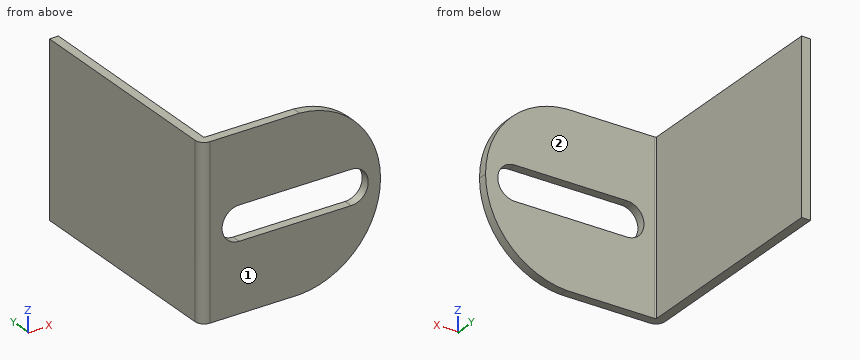
```python
from build123d import *

# Parameters (mm, degrees)
SKETCH1_W           = 19
SKETCH1_H           = 2
BOSS_EXTRUDE1_DEPTH = 38
CUT_EXTRUDE1_DEPTH  = 38


with BuildPart() as part:
    # Sketch1 → Boss-Extrude1 (new body)
    with BuildSketch(Plane.XY):
        with BuildLine():
            ThreePointArc((-18.000000186, -22.8), (-17.941421543, -22.941421356), (-17.800000186, -23))
            Line((-17.800000186, -23), (1.000000186, -23))
            Line((1.000000186, -23), (1.000000186, -25))
            Line((1.000000186, -25), (-18.000000186, -25))
            ThreePointArc((-18.000000186, -25), (-19.414213749, -24.414213562), (-20.000000186, -23))
            Line((-20.000000186, -23), (-20.000000186, 23))
            Line((-20.000000186, 23), (-20.000000186, 25))
            Line((-20.000000186, 25), (-18.000000186, 25))
            Line((-18.000000186, 25), (-18.000000186, 23))
            Line((-18.000000186, 23), (-18.000000186, -22.8))
        make_face()
        with Locations((10.500000186, -24)):
            Rectangle(SKETCH1_W, SKETCH1_H)
    extrude(amount=BOSS_EXTRUDE1_DEPTH)

    # Sketch2 → Cut-Extrude1 (cut)
    with BuildSketch(Plane.XZ.offset(25)):
        with BuildLine():
            Line((20.000000186, 0), (20.000000186, 19))
            ThreePointArc((20.000000186, 19), (14.768114469, 5.896541545), (1.950000354, 0))
            Line((1.950000354, 0), (20.000000186, 0))
        make_face()
        with BuildLine():
            Line((20.000000186, 38), (1.950000354, 38))
            ThreePointArc((1.950000354, 38), (14.768114469, 32.103458455), (20.000000186, 19))
            Line((20.000000186, 19), (20.000000186, 38))
        make_face()
        with BuildLine():
            Line((13.470634361, 22.80060415), (-11.520634006, 22.80060415))
            ThreePointArc((-11.520634006, 22.80060415), (-15.321238156, 19), (-11.520634006, 15.19939585))
            Line((-11.520634006, 15.19939585), (13.470634361, 15.19939585))
            ThreePointArc((13.470634361, 15.19939585), (17.27123851, 19), (13.470634361, 22.80060415))
        make_face()
    extrude(amount=-CUT_EXTRUDE1_DEPTH, mode=Mode.SUBTRACT)


solid = part.part
```
Model file for the job. Use its own axes, mm. Face numbers are marked on the shaded views. A direction names the side the tool comes from. Coordinates: 2 decimals unless noted, no trailing zeros. Write each loop counter-clockwise with the first axis right and the second up, starting at its lowest first coordinate (ties: lowest second). Pieces come first, ordered by that corner, then holes. Notation, with made-up numbers: (-0.75, 32) - (16.25, 32) arc R16 ccw to (16.25, 54) - close; hole circle Ø2 at (82.25, 48.25). An arc over 180 degrees is marked (long way). One line per question, with ' | ' between items. Start each with the question number.
Q1. 3-axis set-ups, long thin cutter, end or side, ignore diameter. For the marked faces 1 and 2: which of +Z, -Z, +X, -X, +Y, -Y reach the whole face in a straight line?
Q2. Cut at A-A, the plane x = -5. List the corners of the cut face in (y, z).
Q3. Pin check, flat tip, straight feed: pin 1 (6 mm diameter, centred on y = 0.5, z = 9, fed in from +X). Stop position of the tip, or through.
Q4. Drill centre lines: line 1 (Y direction, x = 10.5, z = 23); line 2 (X direction, y = -8.5, z = 6.5). Where is each one in solid material? Low to high. Write a range as [from, to].
Q5. Cut at B-B, the plane z = 6. List the corners of the cut face in (x, y).
Q6. Cut at C-C, the plane y = 10. List the corners of the cut face in (x, z).
Q7. Cut at D-D, the plane x = 12.5. List the corners of the cut face in (y, z), then the cut area to 3 significant figures.
Answer below:
1) face 1: +Z, -Z, +X, -X, -Y | face 2: +Z, -Z, +X, +Y
2) outline: (-25, 0) - (-23, 0) - (-23, 15.2) - (-25, 15.2) - close; (-25, 22.8) - (-23, 22.8) - (-23, 38) - (-25, 38) - close
3) pin 1: x = -18
4) line 1: [-25, -23] | line 2: [-20, -18]
5) outline: (-20, -23) arc R2 ccw to (-18, -25) - (14.87, -25) - (14.87, -23) - (-17.8, -23) arc R0.2 cw to (-18, -22.8) - (-18, 25) - (-20, 25) - close
6) outline: (-20, 0) - (-18, 0) - (-18, 38) - (-20, 38) - close
7) outline: (-25, 3.86) - (-23, 3.86) - (-23, 15.2) - (-25, 15.2) - close; (-25, 22.8) - (-23, 22.8) - (-23, 34.14) - (-25, 34.14) - close | area: 45.3 mm^2
